```python
from build123d import *

# Parameters (mm, degrees)
SKETCH1_W           = 50.8
SKETCH1_H           = 36.4998
SKETCH1_W_2         = 46.203262774
SKETCH1_H_2         = 31.7754
BOSS_EXTRUDE1_DEPTH = 36.4998
SKETCH8_R           = 15.748
BOSS_EXTRUDE3_DEPTH = 46.0756
SKETCH9_R           = 5.5499
CUT_EXTRUDE1_DEPTH  = 25.4
CUT_EXTRUDE2_REACH  = 38.5
SKETCH10_R          = 1.27


with BuildPart() as part:
    # Sketch1 → Boss-Extrude1 (new body)
    with BuildSketch(Plane.XY):
        with Locations((25.4, 18.2499)):
            Rectangle(SKETCH1_W, SKETCH1_H)
        with Locations((25.463831387, 18.2499)):
            Rectangle(SKETCH1_W_2, SKETCH1_H_2, mode=Mode.SUBTRACT)
    extrude(amount=BOSS_EXTRUDE1_DEPTH)

    # Sketch8 → Boss-Extrude3 (add)
    with BuildSketch(Plane(origin=(2.3622, 0, 0), x_dir=(0, 0, -1), z_dir=(1, 0, 0))):
        with Locations((-18.2499, 18.2499)):
            Circle(SKETCH8_R)
    extrude(amount=BOSS_EXTRUDE3_DEPTH)

    # Sketch9 → Cut-Extrude1 (cut)
    with BuildSketch(Plane.ZY):
        with Locations((18.2499, 18.2499)):
            Circle(SKETCH9_R)
    extrude(amount=-CUT_EXTRUDE1_DEPTH, mode=Mode.SUBTRACT)

    # Sketch10 → Cut-Extrude2 (cut, up to next)
    with BuildSketch(Plane(origin=(0, 36.4998, 0), x_dir=(1, 0, 0), z_dir=(0, 1, 0)), mode=Mode.PRIVATE) as cut_extrude2_sk1:
        with Locations((38.1, -9.12495)):
            Circle(SKETCH10_R)
    cut_extrude2_tool1 = extrude(cut_extrude2_sk1.sketch, amount=-CUT_EXTRUDE2_REACH, mode=Mode.PRIVATE) & part.part
    add(cut_extrude2_tool1.solids().sort_by_distance((38.1, 36.4998, 9.12495))[0], mode=Mode.SUBTRACT)
    # Sketch10 → Cut-Extrude2 (cut, up to next)
    with BuildSketch(Plane(origin=(0, 36.4998, 0), x_dir=(1, 0, 0), z_dir=(0, 1, 0)), mode=Mode.PRIVATE) as cut_extrude2_sk2:
        with Locations((12.7, -9.12495)):
            Circle(SKETCH10_R)
    cut_extrude2_tool2 = extrude(cut_extrude2_sk2.sketch, amount=-CUT_EXTRUDE2_REACH, mode=Mode.PRIVATE) & part.part
    add(cut_extrude2_tool2.solids().sort_by_distance((12.7, 36.4998, 9.12495))[0], mode=Mode.SUBTRACT)
    # Sketch10 → Cut-Extrude2 (cut, up to next)
    with BuildSketch(Plane(origin=(0, 36.4998, 0), x_dir=(1, 0, 0), z_dir=(0, 1, 0)), mode=Mode.PRIVATE) as cut_extrude2_sk3:
        with Locations((38.1, -27.37485)):
            Circle(SKETCH10_R)
    cut_extrude2_tool3 = extrude(cut_extrude2_sk3.sketch, amount=-CUT_EXTRUDE2_REACH, mode=Mode.PRIVATE) & part.part
    add(cut_extrude2_tool3.solids().sort_by_distance((38.1, 36.4998, 27.37485))[0], mode=Mode.SUBTRACT)
    # Sketch10 → Cut-Extrude2 (cut, up to next)
    with BuildSketch(Plane(origin=(0, 36.4998, 0), x_dir=(1, 0, 0), z_dir=(0, 1, 0)), mode=Mode.PRIVATE) as cut_extrude2_sk4:
        with Locations((12.7, -27.37485)):
            Circle(SKETCH10_R)
    cut_extrude2_tool4 = extrude(cut_extrude2_sk4.sketch, amount=-CUT_EXTRUDE2_REACH, mode=Mode.PRIVATE) & part.part
    add(cut_extrude2_tool4.solids().sort_by_distance((12.7, 36.4998, 27.37485))[0], mode=Mode.SUBTRACT)


solid = part.part
```
Verification items for the finished model (mm, model axes). A direction names the side the tool comes from. Round coordinates to 2 decimals unless told otherwise and drop trailing zeros. Loops run counter-clockwise (first coordinate to the right, second up) from the corner with the lowest first, then second, coordinate; pieces in that order, holes last. Notation, with made-up numbers: (-13, 10) -> (30, 10) arc R23 cw to (30, 19) -> close; hole circle Ø5 at (-9, 56). An arc over 180 degrees is marked (long way). Answer as a JSON object with one key per item and string values.
Q1. Scan lines: line 1 (Z direction, x = 38.1, y = 36); line 2 (Y direction, x = 24, z = 22); line 3 (X direction, y = 15, z = 34.5). Record each from-to range of solid material in increasing order. Write a range as from..to.
Data:
{"line 1": "z = 0..7.85, 10.39..26.1, 28.64..36.5", "line 2": "y = 0..2.36, 2.95..14.16, 22.34..33.54, 34.14..36.5", "line 3": "x = 0..2.36, 48.57..50.8"}
Q2. Go/stop test with flat-tipped pins: P1, Ø5, axis at x = 29, y = 29.5, coming from the +Z side; P2, Ø1, axis at x = 27.5, y = 15.5, coming from the +Z side. Record where each tip stops, or that it passes through.
Data:
{"P1": "stops at z = 31.34", "P2": "stops at z = 33.84"}
Q3. Access from +Z, -Z, +X, -X, +Y, -Y to the whole of each face (thin tool, end or side, straight path). Record for faces 5 (the flat face through (2.362, 7, 6)), 6 (the cylindrical face through (12.52, 12.83, 17.05)), 7 (the flat face through (25, 34.138, 14)), 8 (the cylindrical face through (13.873, 35.335, 27.861)).
Data:
{"face 5": "none", "face 6": "-X", "face 7": "+Z, -Z", "face 8": "+Y"}
Q4. Section check B-B (y = 29). Record the boundary of the cut face in (x, z).
Data:
{"outline": "(0, 0) -> (2.36, 0) -> (2.36, 6.74) -> (48.44, 6.74) -> (48.44, 29.76) -> (2.36, 29.76) -> (2.36, 36.5) -> (0, 36.5) -> close; (48.57, 0) -> (50.8, 0) -> (50.8, 36.5) -> (48.57, 36.5) -> close"}
Q5. Draft check along X on faces 1 (the cylindrical face through (13.873, 35.335, 9.611)), 2 (the flat face through (50.8, 18, 18)), 3 (the flat face through (25.4, 18, 18)), 4 (the flat face through (25, 0, 18)). Enter one of: pulls with the +X half, pulls with the -X half, needs draft (parallel to the pull), parting line crosses it, or undercut.
Data:
{"face 1": "undercut", "face 2": "pulls with the +X half", "face 3": "pulls with the -X half", "face 4": "needs draft"}
Q6. Section check A-A (x = 4). Record the boundary of the cut face in (y, z).
Data:
{"outline": "(0, 0) -> (2.36, 0) -> (2.36, 36.5) -> (0, 36.5) -> close; circle Ø31.5 at (18.25, 18.25); (34.14, 0) -> (36.5, 0) -> (36.5, 36.5) -> (34.14, 36.5) -> close; hole circle Ø11.1 at (18.25, 18.25)"}
Q7. Section check D-D (z = 20). Record the boundary of the cut face in (x, y), then the cut area to 3 significant figures.
Data:
{"outline": "(0, 0) -> (50.8, 0) -> (50.8, 36.5) -> (0, 36.5) -> (0, 23.52) -> (25.4, 23.52) -> (25.4, 12.98) -> (0, 12.98) -> close; hole (2.36, 2.36) -> (48.57, 2.36) -> (48.57, 34.14) -> (2.36, 34.14) -> (2.36, 33.9) -> (48.44, 33.9) -> (48.44, 2.6) -> (2.36, 2.6) -> close", "area": "1,560 mm2"}
Q8. Section check C-C (x = 12.7). Record the boundary of the cut face in (y, z), then the cut area to 3 significant figures.
Data:
{"outline": "(0, 0) -> (2.36, 0) -> (2.36, 36.5) -> (0, 36.5) -> close; circle Ø31.5 at (18.25, 18.25); (34.14, 0) -> (36.5, 0) -> (36.5, 7.85) -> (34.14, 7.85) -> close; (34.14, 10.39) -> (36.5, 10.39) -> (36.5, 26.1) -> (34.14, 26.1) -> close; (34.14, 28.64) -> (36.5, 28.64) -> (36.5, 36.5) -> (34.14, 36.5) -> close; hole circle Ø11.1 at (18.25, 18.25)", "area": "843 mm2"}
